```python
from build123d import *

# Parameters (mm, degrees)
SKETCH1_R           = 200
SKETCH1_R_2         = 30
BOSS_EXTRUDE1_DEPTH = 50
BOSS_EXTRUDE2_START = -11
SKETCH2_R           = 220
SKETCH2_R_2         = 30
BOSS_EXTRUDE2_DEPTH = 11
CUT_EXTRUDE1_DEPTH  = 327.802692767


with BuildPart() as part:
    # Sketch1 → Boss-Extrude1 (new, symmetric)
    with BuildSketch(Plane.XY):
        Circle(SKETCH1_R)
        Circle(SKETCH1_R_2, mode=Mode.SUBTRACT)
    extrude(amount=BOSS_EXTRUDE1_DEPTH, both=True)

    # Sketch2 → Boss-Extrude2 (add)
    with BuildSketch(Plane.XY.offset(50).offset(BOSS_EXTRUDE2_START)):
        Circle(SKETCH2_R)
        Circle(SKETCH2_R_2, mode=Mode.SUBTRACT)
    boss_extrude2 = extrude(amount=BOSS_EXTRUDE2_DEPTH)

    # Mirror1: Boss-Extrude2 across plane
    add(boss_extrude2.mirror(Plane.XY))

    # Sketch3 → Cut-Extrude1 (cut, through all)
    with BuildSketch(Plane.XY.offset(50)):
        with BuildLine():
            Line((9, 19.456611091), (9, 35.88871689))
            ThreePointArc((9, 35.88871689), (0, 37), (-9, 35.88871689))
            Line((-9, 35.88871689), (-9, 19.456611091))
            Line((-9, 19.456611091), (9, 19.456611091))
        make_face()
    extrude(amount=-CUT_EXTRUDE1_DEPTH, mode=Mode.SUBTRACT)


solid = part.part
```
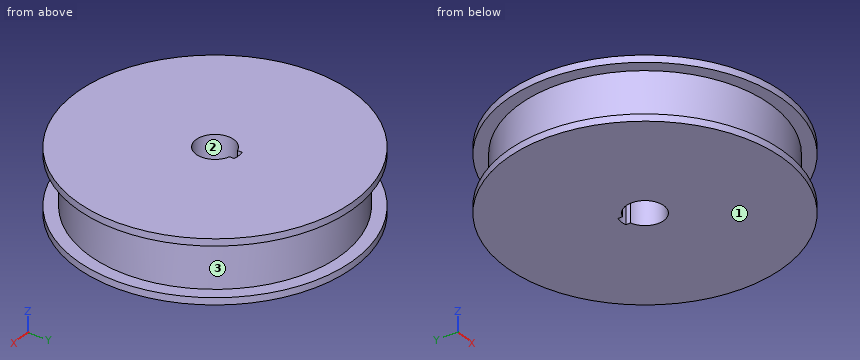
The listing builds one solid part. Answer for the finished solid, in the listing's coordinates (mm). Face numbers are marked on the shaded views. Round coordinates to 2 decimals unless told otherwise and drop trailing zeros. Loops run counter-clockwise (first coordinate to the right, second up) from the corner with the lowest first, then second, coordinate; pieces in that order, holes last.
Q1. Section A-A, the plane y = 0 is taken. Determine the outline of the cut face in (x, z), then the cut area to 3 significant figures.
Q2. For a pull along X with two mould halves and no side action, classify the marked faces 1, 2 and 3 as released by +X, released by -X, zero draft, split by the parting line, or undercut.
Q3. Section C-C, the plane z = -20.5 is taken. Determine the outline of the cut face in (x, y).
Q4. Given pin 1 Ø3 at (y, z) = (104.5, -17) entering from +X; pin 2 Ø1.5 at (x, z) = (102.5, -11) entering from -Y; pin 3 Ø1 at (x, z) = (73, -36.5) entering from -Y, each flat-ended and moving along its own axis, determine where each tip first touches the part or whether it passes through.
Q5. Find the intervals of material crossed by line 1 (Y direction, x = 0, z = 1.5); line 2 (Z direction, x = 172, y = 109); line 3 (Y direction, x = 19.5, z = -8), in increasing order.
Q6. Section B-B, the plane x = 0 is taken. Determine the outline of the cut face in (y, z), then the cut area to 3 significant figures.
Q7. Section D-D, the plane y = -137.5 is taken. Determine the outline of the cut face in (x, z).
Completed:
1. outline: (-220, -50) - (-30, -50) - (-30, 50) - (-220, 50) - (-220, 39) - (-200, 39) - (-200, -39) - (-220, -39) - close; (30, -50) - (220, -50) - (220, -39) - (200, -39) - (200, 39) - (220, 39) - (220, 50) - (30, 50) - close
1. area: 34,900 mm2
2. face 1: zero draft
2. face 2: undercut
2. face 3: split by the parting line
3. outline: circle Ø400 at (0, 0); hole (-9, 28.62) arc R30 ccw (long way) to (9, 28.62) - (9, 35.89) arc R37 ccw to (-9, 35.89) - close
4. pin 1: stops at x = 171.44
4. pin 2: stops at y = -172.18
4. pin 3: stops at y = -186.4
5. line 1: y = -200 to -30, 37 to 200
5. line 2: z = -50 to -39, 39 to 50
5. line 3: y = -199.05 to -22.8, 22.8 to 199.05
6. outline: (-220, -50) - (-30, -50) - (-30, 50) - (-220, 50) - (-220, 39) - (-200, 39) - (-200, -39) - (-220, -39) - close; (37, -50) - (220, -50) - (220, -39) - (200, -39) - (200, 39) - (220, 39) - (220, 50) - (37, 50) - close
6. area: 34,200 mm2
7. outline: (-171.74, -50) - (171.74, -50) - (171.74, -39) - (145.24, -39) - (145.24, 39) - (171.74, 39) - (171.74, 50) - (-171.74, 50) - (-171.74, 39) - (-145.24, 39) - (-145.24, -39) - (-171.74, -39) - close
